from build123d import *

# Parameters (mm, degrees)
F1_R          = 8.89
F1_R_2        = 5.969
F3_R          = 8.89
F3_R_2        = 7.62
F4_DEPTH      = 7.62
F5_DEPTH      = 25.4
F5_DEPTH_BACK = 25.4
F6_R          = 7.62
F7_R          = 7.62
F8_DEPTH      = 38.1
F0_W          = 25.4
F0_H          = 12.7
F9_DEPTH      = 8.89
F9_DEPTH_BACK = 8.89
F10_DEPTH     = 25.4
F11_DEPTH     = 38.1


with BuildPart() as f2:
    # F2: sweep along a path in F0
    with BuildLine(Plane.XY) as f2_path:
        Line((0, 0), (0, 124.469906))
        ThreePointArc((0, 124.469906), (12.7, 137.169906), (25.4, 124.469906))
        Line((25.4, 124.469906), (25.4, 0))
    # F1 (on Front) → F2 (sweep)
    with BuildSketch(Plane.XZ):
        Circle(F1_R)
        Circle(F1_R_2, mode=Mode.SUBTRACT)
    sweep(path=f2_path.line)

    # F3 (on face) → F4 (cut)
    with BuildSketch(Plane.XZ):
        Circle(F3_R)
        Circle(F3_R_2, mode=Mode.SUBTRACT)
        with BuildLine():
            ThreePointArc((34.29, 0), (25.4, 8.89), (16.51, 0))
            ThreePointArc((16.51, 0), (25.4, -8.89), (34.29, 0))
        make_face()
        with BuildLine():
            ThreePointArc((33.02, 0), (25.4, -7.62), (17.78, 0))
            ThreePointArc((17.78, 0), (25.4, 7.62), (33.02, 0))
        make_face(mode=Mode.SUBTRACT)
    extrude(amount=-F4_DEPTH, mode=Mode.SUBTRACT)

    # F0 (on Top) → F5 (cut, two sides)
    with BuildSketch(Plane.XY) as f5_sk:
        with BuildLine():
            Line((-27.3511596024, 56.5561708785), (0, 56.5561708785))
            Line((0, 56.5561708785), (0, 124.469906))
            ThreePointArc((0, 124.469906), (3.7197438789, 133.4501621211), (12.7, 137.169906))
            ThreePointArc((12.7, 137.169906), (21.6802561211, 133.4501621211), (25.4, 124.469906))
            Line((25.4, 124.469906), (25.4, 56.5561708785))
            Line((25.4, 56.5561708785), (45.1116599143, 56.5561708785))
            Line((45.1116599143, 56.5561708785), (45.1116599143, 146.6434597969))
            Line((45.1116599143, 146.6434597969), (-27.3511596024, 146.6434597969))
            Line((-27.3511596024, 146.6434597969), (-27.3511596024, 56.5561708785))
        make_face()
        with BuildLine():
            Line((0, 124.469906), (0, 56.5561708785))
            Line((0, 56.5561708785), (12.7, 56.5561708785))
            Line((12.7, 56.5561708785), (12.7, 137.169906))
            ThreePointArc((12.7, 137.169906), (3.7197438789, 133.4501621211), (0, 124.469906))
        make_face()
        with BuildLine():
            Line((12.7, 56.5561708785), (25.4, 56.5561708785))
            Line((25.4, 56.5561708785), (25.4, 124.469906))
            ThreePointArc((25.4, 124.469906), (21.6802561211, 133.4501621211), (12.7, 137.169906))
            Line((12.7, 137.169906), (12.7, 56.5561708785))
        make_face()
    extrude(amount=-F5_DEPTH, mode=Mode.SUBTRACT)
    extrude(f5_sk.sketch, amount=F5_DEPTH_BACK, mode=Mode.SUBTRACT)

    # F6 (on face) + F7 (on face) → F8 (cut)
    with BuildSketch(Plane(origin=(0, 56.5561708785, 0), x_dir=(-1, 0, 0), z_dir=(0, 1, 0))):
        with Locations((-25.4, 0)):
            Circle(F6_R)
    with BuildSketch(Plane(origin=(0, 56.5561708785, 0), x_dir=(-1, 0, 0), z_dir=(0, 1, 0))):
        Circle(F7_R)
    extrude(amount=-F8_DEPTH, mode=Mode.SUBTRACT)

    # F0 (on Top) → F9 (join, two sides)
    with BuildSketch(Plane.XY) as f9_sk:
        with Locations((12.7, 34.5915263355)):
            Rectangle(F0_W, F0_H)
    extrude(amount=F9_DEPTH)
    extrude(f9_sk.sketch, amount=-F9_DEPTH_BACK)

    # F7 (on face) + F6 (on face) → F10 (cut)
    with BuildSketch(Plane(origin=(0, 56.5561708785, 0), x_dir=(-1, 0, 0), z_dir=(0, 1, 0))):
        Circle(F7_R)
    with BuildSketch(Plane(origin=(0, 56.5561708785, 0), x_dir=(-1, 0, 0), z_dir=(0, 1, 0))):
        with Locations((-25.4, 0)):
            Circle(F6_R)
    extrude(amount=-F10_DEPTH, mode=Mode.SUBTRACT)

    # F7 (on face) + F6 (on face) → F11 (cut)
    with BuildSketch(Plane(origin=(0, 56.5561708785, 0), x_dir=(-1, 0, 0), z_dir=(0, 1, 0))):
        Circle(F7_R)
    with BuildSketch(Plane(origin=(0, 56.5561708785, 0), x_dir=(-1, 0, 0), z_dir=(0, 1, 0))):
        with Locations((-25.4, 0)):
            Circle(F6_R)
    extrude(amount=-F11_DEPTH, mode=Mode.SUBTRACT)


solid = f2.part
Could you check a few things on this model? Use its own coordinates, in mm. A direction names the side the tool comes from. Give positions to 0.01 mm unless a question says otherwise; leave off trailing zeros. Order: outer loops, then holes, each group sorted by start corner. A loop starts at its lowest first (then second) coordinate and runs counter-clockwise, first axis right, second up. Notation, with made-up numbers: (71, 18) -> (91, 18) arc R11 ccw to (91, 24) -> close; hole circle Ø5 at (23.25, 71.25). An arc over 180 degrees is marked (long way). Answer in a Markdown table with one row per item. Add a question column.
Item 1: Imagine slicing it at B-B (x = 26). List the corners of the cut face in (y, z) for me, and give its area (3 significant figures).
Item 2: Imagine slicing it at D-D (z = 0). Count the separate pieces of the cut face and the enclosed holes in it, and give its area (3 significant figures).
Item 3: For faces 1 (the flat face through (7, 56.556, 4)), 2 (the flat face through (31, 18.456, -3)), 3 (the flat face through (13, 28.242, 0)), which set-ups out of +Z, -Z, +X, -X, +Y, -Y let a thin tool reach every point of the face, with its end or its side?
Item 4: Imagine slicing it at A-A (y = 13). List the corners of the cut face in (x, z) for me.
Item 5: I'm going to push flat-ended pins straight in: P1, Ø1, axis at y = 19.5, z = 3.5, coming from the -X side; P2, Ø1, axis at y = 30.5, z = -5, coming from the +X side; P3, Ø7, axis at x = 0, z = 0, coming from the +Y side; P4, Ø10, axis at x = 18, y = 12, coming from the -Z side. Where does each tip first touch, or does it pass through?
Item 6: Please list where these lines run through material, in increasing order: probe 1 along Z at (x, y) = (0, 7); probe 2 along Z at (x, y) = (25, 37); probe 3 along X at (y, z) = (45.5, 6.75).
Item 7: We'd pull the mould along Z, two halves only. Please class faces 4 (the flat face through (21, 0, -5)), 5 (the cylindrical face through (-8.88, 32.43, -0.39)), 6 (the cylindrical face through (1.65, 37.77, -7.44)): pulls with the +Z half, pulls with the -Z half, needs draft (parallel to the pull), parting line crosses it, or undercut.
Item 8: Imagine slicing it at C-C (x = 18.5). List the corners of the cut face in (y, z) for me.
Result:
| question | item | result |
|---|---|---|
| 1 | outline | (0, -7.6) -> (7.62, -7.6) -> (7.62, -8.87) -> (56.56, -8.87) -> (56.56, -7.6) -> (18.46, -7.6) -> (18.46, -5.94) -> (0, -5.94) -> close; (0, 5.94) -> (18.46, 5.94) -> (18.46, 7.6) -> (56.56, 7.6) -> (56.56, 8.87) -> (7.62, 8.87) -> (7.62, 7.6) -> (0, 7.6) -> close |
| 1 | area | 186 mm2 |
| 2 | separate pieces | 3 |
| 2 | enclosed holes | 0 |
| 2 | area | 467 mm2 |
| 3 | face 1 | +Z, -Z, +X, -X, +Y |
| 3 | face 2 | +Y |
| 3 | face 3 | -Y |
| 4 | outline | circle Ø17.78 at (0, 0); circle Ø17.78 at (25.4, 0); hole circle Ø11.94 at (0, 0); hole circle Ø11.94 at (25.4, 0) |
| 5 | P1 | x = -8.37 |
| 5 | P2 | x = 33.07 |
| 5 | P3 | through |
| 5 | P4 | z = -8.56 |
| 6 | probe 1 | -7.62 to -5.97, 5.97 to 7.62 |
| 6 | probe 2 | -8.89 to -7.61, 7.61 to 8.89 |
| 6 | probe 3 | -5.79 to -3.54, 3.54 to 5.79, 19.61 to 21.86, 28.94 to 31.19 |
| 7 | face 4 | needs draft |
| 7 | face 5 | parting line crosses it |
| 7 | face 6 | undercut |
| 8 | outline | (0, -3.23) -> (7.62, -3.23) -> (7.62, -5.61) -> (28.24, -5.61) -> (28.24, -8.89) -> (40.94, -8.89) -> (40.94, -5.61) -> (56.56, -5.61) -> (56.56, -3.23) -> (18.46, -3.23) -> (18.46, 3.23) -> (56.56, 3.23) -> (56.56, 5.61) -> (40.94, 5.61) -> (40.94, 8.89) -> (28.24, 8.89) -> (28.24, 5.61) -> (7.62, 5.61) -> (7.62, 3.23) -> (0, 3.23) -> close |
